Source: three-view drawing plus pictorial views. Frame: mm from the lowest corner of the part. A direction names the side the tool comes from. Round coordinates to 2 decimals unless told otherwise and drop trailing zeros. Loops run counter-clockwise (first coordinate to the right, second up) from the corner with the lowest first, then second, coordinate; pieces in that order, holes last. Notation, with made-up numbers: (61.25, 43) -> (72.25, 43) arc R16 ccw to (72.25, 74) -> close; hole circle Ø10 at (83, -10.75). An arc over 180 degrees is marked (long way). Answer in a Markdown table with one row per item.
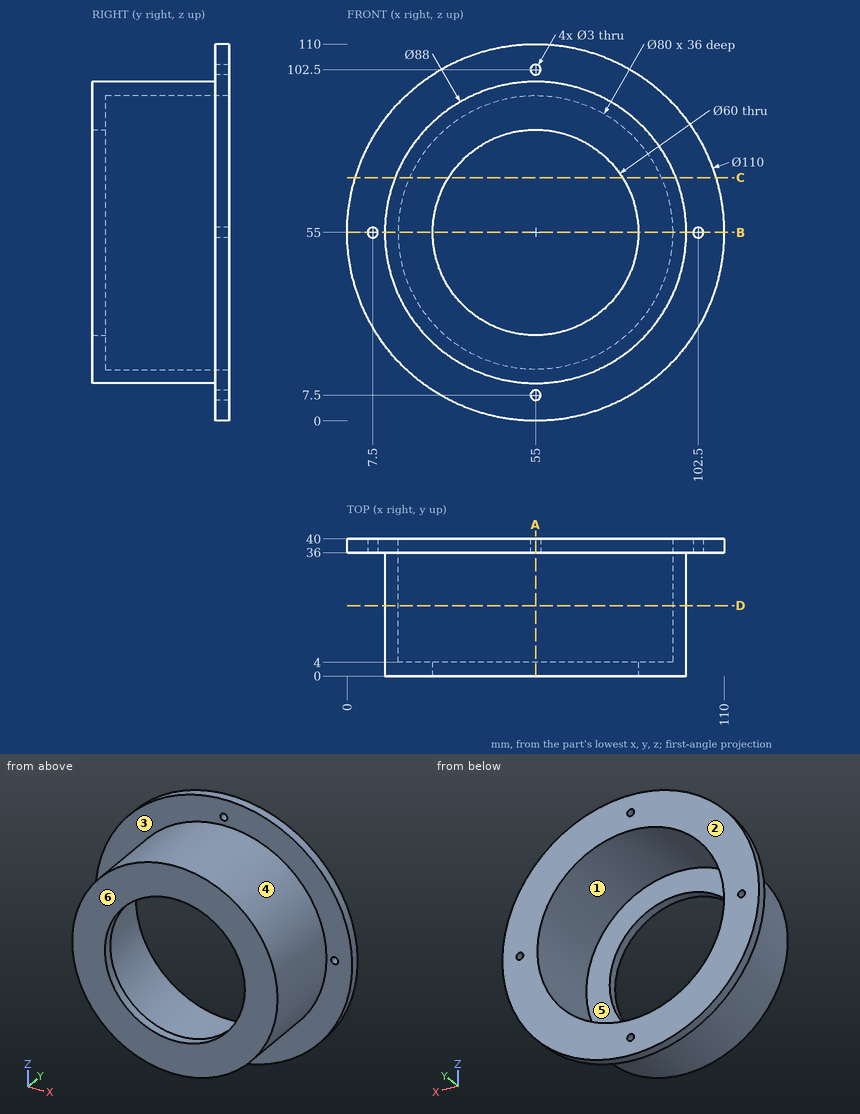
Item 1: Cut plane B-B (z = 55). Output: boundary loops of the cut face in (x, y), then the cut area to 3 significant figures.
Answer:
| item | result |
|---|---|
| outline | (0, 36) -> (6, 36) -> (6, 40) -> (0, 40) -> close; (9, 36) -> (11, 36) -> (11, 0) -> (25, 0) -> (25, 4) -> (15, 4) -> (15, 40) -> (9, 40) -> close; (85, 0) -> (99, 0) -> (99, 36) -> (101, 36) -> (101, 40) -> (95, 40) -> (95, 4) -> (85, 4) -> close; (104, 36) -> (110, 36) -> (110, 40) -> (104, 40) -> close |
| area | 464 mm² |
Item 2: Line query: probe 1 along Z at (x, y) = (55, 18); probe 2 along Y at (x, z) = (18, 55); probe 3 along X at (y, z) = (7, 70). Output: solid intervals per line, ascending. Write a range as [from, to].
Answer:
| item | result |
|---|---|
| probe 1 | z = [11, 15], [95, 99] |
| probe 2 | y = [0, 4] |
| probe 3 | x = [13.64, 17.92], [92.08, 96.36] |
Item 3: Pin query (flat end, axial travel): pin 1 Ø2.5 at (x, z) = (55, 102.5) entering from -Y; pin 2 Ø5 at (x, z) = (55, 7.5) entering from -Y; pin 3 Ø1.5 at (y, z) = (24, 93) entering from +X; pin 4 Ø2 at (x, y) = (78, 15) entering from -Z. Return the tip coordinate at first contact, or that it passes through.
Answer:
| item | result |
|---|---|
| pin 1 | passes through |
| pin 2 | stops at y = 36 |
| pin 3 | stops at x = 78.42 |
| pin 4 | stops at z = 16.89 |
Item 4: Cut plane D-D (y = 20.5). Output: boundary loops of the cut face in (x, z).
Answer:
| item | result |
|---|---|
| outline | circle Ø88 at (55, 55); hole circle Ø80 at (55, 55) |
Item 5: Cut plane C-C (z = 71). Output: boundary loops of the cut face in (x, y), then the cut area to 3 significant figures.
Answer:
| item | result |
|---|---|
| outline | (2.38, 36) -> (14.01, 36) -> (14.01, 0) -> (29.62, 0) -> (29.62, 4) -> (18.34, 4) -> (18.34, 40) -> (2.38, 40) -> close; (80.38, 0) -> (95.99, 0) -> (95.99, 36) -> (107.62, 36) -> (107.62, 40) -> (91.66, 40) -> (91.66, 4) -> (80.38, 4) -> close |
| area | 530 mm² |
Item 6: Cut plane A-A (x = 55). Output: boundary loops of the cut face in (y, z), then the cut area to 3 significant figures.
Answer:
| item | result |
|---|---|
| outline | (0, 11) -> (36, 11) -> (36, 9) -> (40, 9) -> (40, 15) -> (4, 15) -> (4, 25) -> (0, 25) -> close; (0, 85) -> (4, 85) -> (4, 95) -> (40, 95) -> (40, 101) -> (36, 101) -> (36, 99) -> (0, 99) -> close; (36, 0) -> (40, 0) -> (40, 6) -> (36, 6) -> close; (36, 104) -> (40, 104) -> (40, 110) -> (36, 110) -> close |
| area | 464 mm² |
Item 7: Draft query along X for the marked faces 4, 5 and 6. Return one class per face: pulls with the +X half, pulls with the -X half, needs draft (parallel to the pull), parting line crosses it, or undercut.
Answer:
| item | result |
|---|---|
| face 4 | parting line crosses it |
| face 5 | undercut |
| face 6 | needs draft |
Item 8: Reachability of the marked faces 1, 2 and 3 from +Z, -Z, +X, -X, +Y, -Y: full face, straight path, thin tool, end or side. Return the list, or none.
Answer:
| item | result |
|---|---|
| face 1 | +Y |
| face 2 | +Z, -Z, +X, -X, +Y |
| face 3 | -Y |
